Build history of the part. All positions in model axes, mm. Coordinates: 2 decimals unless noted, no trailing zeros. Loops run counter-clockwise (first coordinate to the right, second up) from the corner with the lowest first, then second, coordinate; pieces in that order, holes last.
Item 1: Drill centre lines: line 1 along Z through (x, y) = (2.5, 314); line 2 along Z through (x, y) = (4, 280); line 3 along Y through (x, z) = (8, -40). Where is each one in solid material? Low to high.
Item 2: Flat gauge pins, fed straight in: pin 1 (14.5 mm diameter, centred on y = 280, z = 0, fed in from +X); pin 2 (6 mm diameter, centred on x = 4.5, y = 239.5, fed in from -Z); pin 3 (6 mm diameter, centred on x = 6, y = 117, fed in from +Z). Where does each tip first touch, or does it go through?
Item 3: Cut at B-B (y = 280). List the corners of the cut face in (x, z).
Item 4: Cut at A-A (z = 30). List the corners of the cut face in (x, y), and give its area (3 significant figures).
Item 5: Cut at D-D (z = -114.5). List the corners of the cut face in (x, y).
Item 6: Cut at C-C (x = 7.25). Count the separate pieces of the cut face and the enclosed holes in it, and give its area (3 significant figures).
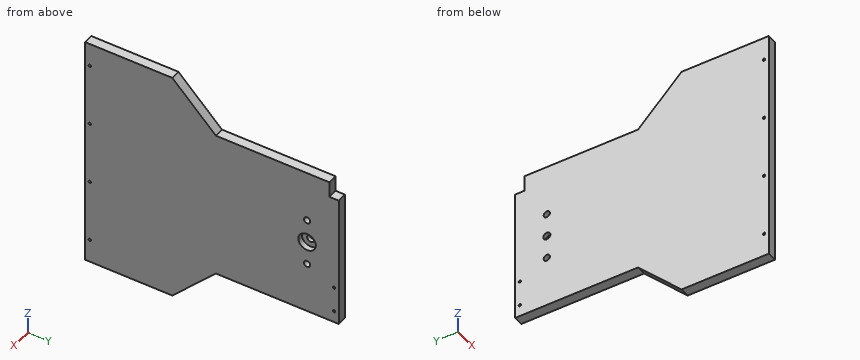
from build123d import *

# Parameters (mm, degrees)
BOSS_EXTRUDE1_DEPTH = 12
SKETCH2_R           = 4
CUT_EXTRUDE1_DEPTH  = 13
SKETCH3_R           = 4.5
CUT_EXTRUDE2_DEPTH  = 13
SKETCH4_R           = 11.05
CUT_EXTRUDE3_DEPTH  = 7
SKETCH5_W           = 20
SKETCH5_H           = 12
CUT_EXTRUDE4_DEPTH  = 13
SKETCH6_R           = 1.55
CUT_EXTRUDE5_DEPTH  = 13


with BuildPart() as part:
    # Sketch1 → Boss-Extrude1 (new body)
    with BuildSketch(Plane(origin=(0, 0, 0), x_dir=(0, 0, -1), z_dir=(1, 0, 0))):
        Polygon((95, 320), (-95, 320), (-95, 165), (-150, 110), (-150, 0), (150, 0), (150, 110), (95, 165), align=None)
    extrude(amount=BOSS_EXTRUDE1_DEPTH)

    # Sketch2 → Cut-Extrude1 (cut, through all)
    with BuildSketch(Plane.ZY):
        with Locations((30, 280)):
            Circle(SKETCH2_R)
        with Locations((-30, 280)):
            Circle(SKETCH2_R)
    extrude(amount=-CUT_EXTRUDE1_DEPTH, mode=Mode.SUBTRACT)

    # Sketch3 → Cut-Extrude2 (cut, through all)
    with BuildSketch(Plane.ZY):
        with Locations((0, 280)):
            Circle(SKETCH3_R)
    extrude(amount=-CUT_EXTRUDE2_DEPTH, mode=Mode.SUBTRACT)

    # Sketch4 → Cut-Extrude3 (cut)
    with BuildSketch(Plane(origin=(12, 0, 0), x_dir=(0, 0, -1), z_dir=(1, 0, 0))):
        with Locations((0, 280)):
            Circle(SKETCH4_R)
    extrude(amount=-CUT_EXTRUDE3_DEPTH, mode=Mode.SUBTRACT)

    # Sketch5 → Cut-Extrude4 (cut, through all)
    with BuildSketch(Plane(origin=(12, 0, 0), x_dir=(0, 0, -1), z_dir=(1, 0, 0))):
        with Locations((-85, 314)):
            Rectangle(SKETCH5_W, SKETCH5_H)
    extrude(amount=-CUT_EXTRUDE4_DEPTH, mode=Mode.SUBTRACT)

    # Sketch6 → Cut-Extrude5 (cut, through all)
    with BuildSketch(Plane(origin=(12, 0, 0), x_dir=(0, 0, -1), z_dir=(1, 0, 0))):
        with Locations((-120, 6)):
            Circle(SKETCH6_R)
        with Locations((-40, 6)):
            Circle(SKETCH6_R)
        with Locations((40, 6)):
            Circle(SKETCH6_R)
        with Locations((120, 6)):
            Circle(SKETCH6_R)
        with Locations((80, 314)):
            Circle(SKETCH6_R)
        with Locations((47.5, 314)):
            Circle(SKETCH6_R)
    extrude(amount=-CUT_EXTRUDE5_DEPTH, mode=Mode.SUBTRACT)


solid = part.part
Filled sheet:
1. line 1: z = -95 to -81.55, -78.45 to -49.05, -45.95 to 75
1. line 2: z = -95 to -34, -26 to -4.5, 4.5 to 26, 34 to 95
1. line 3: y = 0 to 4.45, 7.55 to 320
2. pin 1: stops at x = 5
2. pin 2: stops at z = -95
2. pin 3: stops at z = 146
3. outline: (0, -95) - (12, -95) - (12, -34) - (0, -34) - close; (0, -26) - (12, -26) - (12, -11.05) - (5, -11.05) - (5, -4.5) - (0, -4.5) - close; (0, 4.5) - (5, 4.5) - (5, 11.05) - (12, 11.05) - (12, 26) - (0, 26) - close; (0, 34) - (12, 34) - (12, 95) - (0, 95) - close
4. outline: (0, 0) - (12, 0) - (12, 276) - (0, 276) - close; (0, 284) - (12, 284) - (12, 320) - (0, 320) - close
4. area: 3,740 mm2
5. outline: (0, 0) - (12, 0) - (12, 145.5) - (0, 145.5) - close
6. separate pieces: 1
6. enclosed holes: 9
6. area: 75,200 mm2
